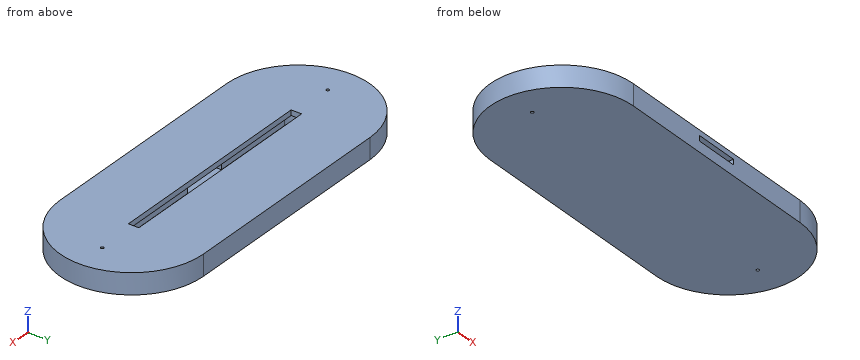
```python
from build123d import *

# Parameters (mm, degrees)
PAD_DEPTH          = 9
POCKET_DEPTH       = 6
SKETCH002_W        = 26.5
SKETCH002_H        = 35
POCKET001_DEPTH    = 6
SKETCH003_W        = 127
SKETCH003_H        = 6
PAD001_DEPTH       = 3
SKETCH004_R        = 0.85
POCKET002_DEPTH    = 467.245989
POLARPATTERN_COUNT = 2
SKETCH005_W        = 26.5
SKETCH005_H        = 7.5
PAD002_DEPTH       = 3


with BuildPart() as part:
    # Sketch → Pad (new body)
    with BuildSketch(Plane.XY):
        with BuildLine():
            ThreePointArc((-65, 41), (-106, 0), (-65, -41))
            Line((-65, -41), (65, -41))
            ThreePointArc((65, -41), (106, 0), (65, 41))
            Line((-65, 41), (65, 41))
        make_face()
    extrude(amount=PAD_DEPTH)

    # Sketch001 (on Face6 of Pad) → Pocket (cut)
    with BuildSketch(Plane.XY.offset(9)):
        with BuildLine():
            ThreePointArc((-62.5, 6), (-68.5, 0), (-62.5, -6))
            Line((-62.5, -6), (62.5, -6))
            ThreePointArc((62.5, -6), (68.5, 0), (62.5, 6))
            Line((-62.5, 6), (62.5, 6))
        make_face()
    extrude(amount=-POCKET_DEPTH, mode=Mode.SUBTRACT)

    # Sketch002 (on Face5 of Pocket) → Pocket001 (cut)
    with BuildSketch(Plane.XY.offset(9)):
        with Locations((0, -23.5)):
            Rectangle(SKETCH002_W, SKETCH002_H)
    extrude(amount=-POCKET001_DEPTH, mode=Mode.SUBTRACT)

    # Sketch003 (on Face5 of Pocket001) → Pad001 (join)
    with BuildSketch(Plane.XY.offset(9)):
        with BuildLine():
            ThreePointArc((-65, 41), (-106, 0), (-65, -41))
            Line((-65, -41), (65, -41))
            ThreePointArc((65, -41), (106, 0), (65, 41))
            Line((-65, 41), (65, 41))
        make_face()
        Rectangle(SKETCH003_W, SKETCH003_H, mode=Mode.SUBTRACT)
    extrude(amount=PAD001_DEPTH)

    # Sketch004 (on Face12 of Pad001) → Pocket002 (cut, through all)
    with BuildSketch(Plane.XY.offset(12)):
        with Locations((-88, 0)):
            Circle(SKETCH004_R)
    pocket002 = extrude(amount=-POCKET002_DEPTH, mode=Mode.SUBTRACT)

    # PolarPattern: Pocket002 ×2 about axis
    polarpattern_axis = Axis((0, 0, 12), (0, 0, 1))
    for i in range(1, POLARPATTERN_COUNT):
        add(pocket002.rotate(polarpattern_axis, i * 360 / POLARPATTERN_COUNT), mode=Mode.SUBTRACT)

    # Sketch005 (on Face10 of PolarPattern) → Pad002 (join)
    with BuildSketch(Plane.XY.offset(3)):
        with Locations((0, -37.25)):
            Rectangle(SKETCH005_W, SKETCH005_H)
    extrude(amount=PAD002_DEPTH)


solid = part.part
```
Design review of the part built by this model. Coordinates are the model's own, in mm. Coordinates: 2 decimals unless noted, no trailing zeros. Order: outer loops, then holes, each group sorted by start corner. A loop starts at its lowest first (then second) coordinate and runs counter-clockwise, first axis right, second up.
1) Take a section at D-D, the plane y = 20. Give the boundary of the cut face in (x, z).
2) Wall thickness on line 1 along Y through (x, z) = (-9.5, 10); line 2 along Y through (x, z) = (-47, 3.5); line 3 along Z through (x, y) = (-65.5, -2): over which ranges is each line inside the solid? List them lowest first.
3) Take a section at A-A, the plane x = 8. Give the boundary of the cut face in (y, z).
4) Take a section at B-B, the plane y = -20. Give the boundary of the cut face in (x, z).
5) Clearance check with flat-ended pins moving along their axes: pin 1 (6 mm diameter, centred on y = -15.5, z = 10, fed in from -X); pin 2 (3 mm diameter, centred on x = -67, z = 3, fed in from +Y); pin 3 (5 mm diameter, centred on y = -19, z = 4, fed in from -X). State where each tip first meets the part, or that it passes through.
6) Take a section at C-C, the plane x = -20.5. Give the boundary of the cut face in (y, z), and give its area (3 significant figures).
Returned:
1. outline: (-100.79, 0) - (100.79, 0) - (100.79, 12) - (-100.79, 12) - close
2. line 1: y = -41 to -3, 3 to 41
2. line 2: y = -41 to -6, 6 to 41
2. line 3: z = 0 to 3, 9 to 12
3. outline: (-41, 0) - (41, 0) - (41, 12) - (3, 12) - (3, 9) - (6, 9) - (6, 3) - (-33.5, 3) - (-33.5, 6) - (-41, 6) - close; (-41, 9) - (-3, 9) - (-3, 12) - (-41, 12) - close
4. outline: (-100.79, 0) - (100.79, 0) - (100.79, 12) - (-100.79, 12) - close; hole (-13.25, 3) - (13.25, 3) - (13.25, 9) - (-13.25, 9) - close
5. pin 1: stops at x = -104.05
5. pin 2: stops at y = 41
5. pin 3: stops at x = -102.53
6. outline: (-41, 0) - (41, 0) - (41, 12) - (3, 12) - (3, 9) - (6, 9) - (6, 3) - (-6, 3) - (-6, 9) - (-3, 9) - (-3, 12) - (-41, 12) - close
6. area: 894 mm2
